For this review, use the dimensioned drawing (mm, ordinates from the lowest corner) and the shaded views. A direction names the side the tool comes from. Coordinates: 2 decimals unless noted, no trailing zeros. Loops run counter-clockwise (first coordinate to the right, second up) from the corner with the lowest first, then second, coordinate; pieces in that order, holes last. Notation, with made-up numbers: (77, -28) -> (129, -28) arc R22 ccw to (129, 2) -> close; hole circle Ø9 at (-0.5, 83). An arc over 180 degrees is marked (long way). One line per question, with ' | ' between items. Start each with the question number.
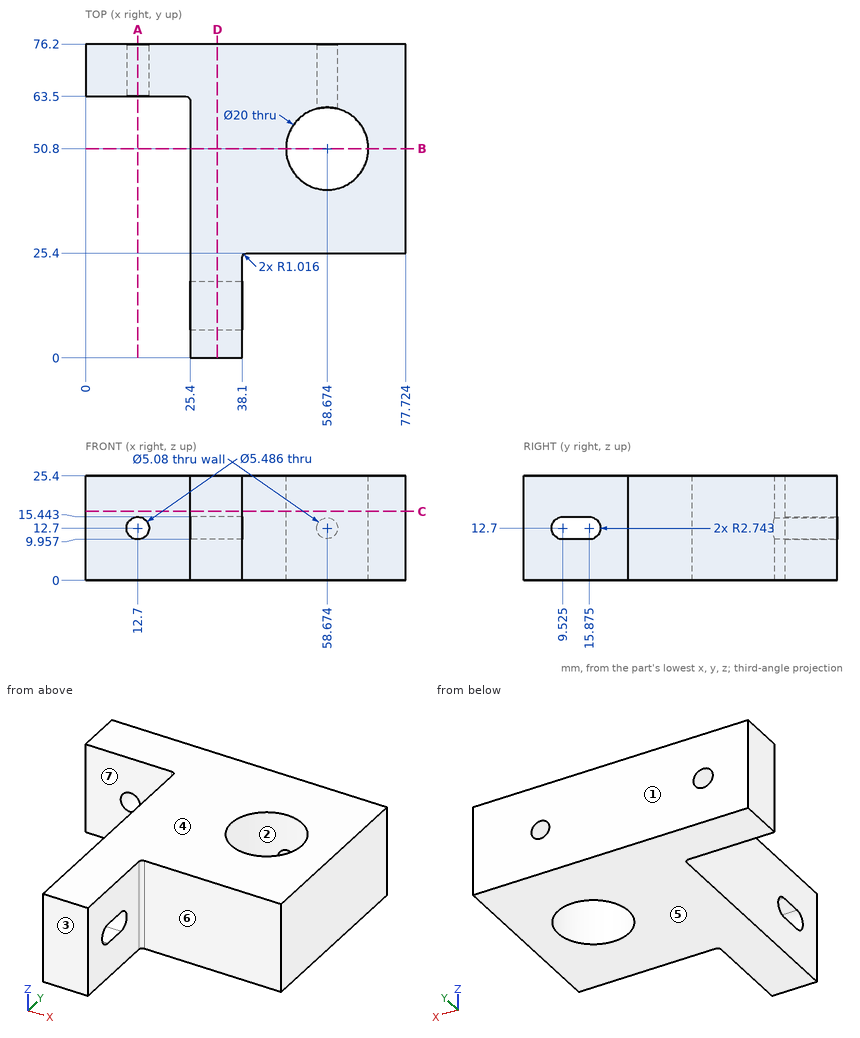
1) Insertion check: pin 1 Ø7.5 at (y, z) = (9.5, 9.5) entering from +X; pin 2 Ø7.5 at (x, z) = (6, 8) entering from -Y; pin 3 Ø10 at (y, z) = (22.5, 5) entering from +X; pin 4 Ø3 at (y, z) = (15, 7) entering from -X. Each pin has a flat end and moves straight along its axis. Give the tip position at first contact, or say it passes through.
2) Machinability: for the marked faces 5, 6 and 7, which of the approach directions +Z, -Z, +X, -X, +Y, -Y give a long, thin tool a straight path to every point of the face, cutting with its end or side? Answer none if there is none.
3) Consider section B-B, the plane y = 50.8. Write out the cut boundary in (x, z), plus the area to 3 significant figures.
4) Consider section A-A, the plane x = 12.7. Write out the cut boundary in (y, z), plus the area to 3 significant figures.
5) Consider section C-C, the plane z = 16.75. Write out the cut boundary in (x, y), plus the area to 3 significant figures.
6) Wall thickness on L1, parallel to X at y = 7.5, z = 4.25; L2, parallel to Y at x = 48.5, z = 5.5; L3, parallel to Y at x = 59.5, z = 20.25 (1 decimal): over which ranges is each line inside the solid? List them lowest first.
7) Consider section D-D, the plane x = 32. Write out the cut boundary in (y, z) (1 decimal).
8) Mouldability with a two-part tool opening along Y and no side actions: class the marked faces 1, 2, 3 and 4 as +Y half, -Y half, draft (parallel to the pull), parting line (faces both ways), or undercut.
Filled sheet:
1) pin 1: x = 38.1 | pin 2: y = 63.5 | pin 3: x = 77.72 | pin 4: x = 25.4
2) face 5: -Z, +X, -X, +Y, -Y | face 6: +Z, -Z, +X, -Y | face 7: +Z, -Z, -X, -Y
3) outline: (25.4, 0) -> (48.67, 0) -> (48.67, 25.4) -> (25.4, 25.4) -> close; (68.67, 0) -> (77.72, 0) -> (77.72, 25.4) -> (68.67, 25.4) -> close | area: 821 mm^2
4) outline: (63.5, 0) -> (76.2, 0) -> (76.2, 9.96) -> (63.5, 9.96) -> close; (63.5, 15.44) -> (76.2, 15.44) -> (76.2, 25.4) -> (63.5, 25.4) -> close | area: 253 mm^2
5) outline: (0, 63.5) -> (24.38, 63.5) arc R1.02 cw to (25.4, 62.48) -> (25.4, 0) -> (38.1, 0) -> (38.1, 24.38) arc R1.02 cw to (39.12, 25.4) -> (77.72, 25.4) -> (77.72, 76.2) -> (0, 76.2) -> close; hole circle Ø20 at (58.67, 50.8) | area: 2,990 mm^2
6) L1: 25.4 to 38.1 | L2: 25.4 to 76.2 | L3: 25.4 to 40.8, 60.8 to 76.2
7) outline: (0, 0) -> (76.2, 0) -> (76.2, 25.4) -> (0, 25.4) -> close; hole (9.5, 10) -> (15.9, 10) arc R2.7 ccw to (15.9, 15.4) -> (9.5, 15.4) arc R2.7 ccw to start
8) face 1: +Y half | face 2: undercut | face 3: -Y half | face 4: draft
